Verification items for this drawing (mm, ordinates from the low corner). A direction names the side the tool comes from. Round coordinates to 2 decimals unless told otherwise and drop trailing zeros. Order: outer loops, then holes, each group sorted by start corner. A loop starts at its lowest first (then second) coordinate and runs counter-clockwise, first axis right, second up. Notation, with made-up numbers: M -27,27 L 5,27 A30 cw 5,62 Z; hole C 17.25,87 d2. An arc over 180 degrees is marked long. Return JSON: item names as keys, results as strings. Group by question number.
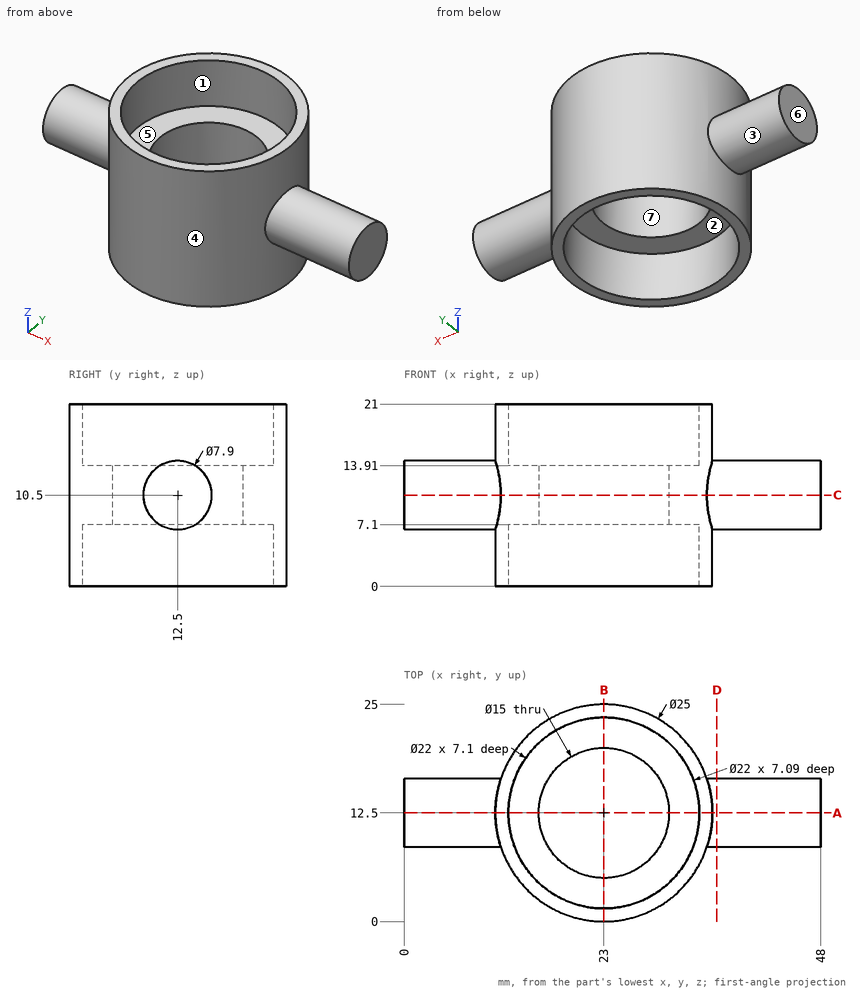
Q1. Section check A-A on y = 12.5. Record the cut outline in (x, z).
Q2. Section check C-C on z = 10.5. Record the cut outline in (x, y).
Q3. Material ranges on line 1 along Y through (x, z) = (23, 18.5); line 2 along Y through (x, z) = (23, 9.5); line 3 along Z through (x, y) = (17, 7), recorded low to high.
Q4. Section check B-B on x = 23. Record the cut outline in (y, z).
Q5. Depth check by flat-ended pin: pin 1 Ø4 at (y, z) = (20, 18.5) entering from +X (3 decimals); pin 2 Ø3 at (x, y) = (39, 13.5) entering from +Z; pin 3 Ø3 at (y, z) = (21, 15) entering from +X. Enter the tip coordinate at first touch or a pass-through.
Q6. Release check for a two-part mould opening along X. For the marked faces 4, 5, 6 and 7 record: +X half, -X half, draft (parallel to the pull), parting line (faces both ways), or undercut.
Q7. Section check D-D on x = 36. Record the cut outline in (y, z).
Q8. Set-up check for the marked faces 1, 2 and 3: record each of +Z, -Z, +X, -X, +Y, -Y from which the full face is reachable in a straight line by a thin tool's end or side.
Geometry check:
{
 "1": {"outline": "M 0,6.55 L 10.5,6.55 L 10.5,0 L 12,0 L 12,7.1 L 15.5,7.1 L 15.5,13.91 L 12,13.91 L 12,21 L 10.5,21 L 10.5,14.45 L 0,14.45 Z; M 30.5,7.1 L 34,7.1 L 34,0 L 35.5,0 L 35.5,6.55 L 48,6.55 L 48,14.45 L 35.5,14.45 L 35.5,21 L 34,21 L 34,13.91 L 30.5,13.91 Z"},
 "2": {"outline": "M 0,8.55 L 11.14,8.55 A12.5 ccw 34.86,8.55 L 48,8.55 L 48,16.45 L 34.86,16.45 A12.5 ccw 11.14,16.45 L 0,16.45 Z; hole C 23,12.5 d15"},
 "3": {"line 1": "y = 0 to 1.5, 23.5 to 25", "line 2": "y = 0 to 5, 20 to 25", "line 3": "z = 7.1 to 13.91"},
 "4": {"outline": "M 0,0 L 1.5,0 L 1.5,7.1 L 5,7.1 L 5,13.91 L 1.5,13.91 L 1.5,21 L 0,21 Z; M 20,7.1 L 23.5,7.1 L 23.5,0 L 25,0 L 25,21 L 23.5,21 L 23.5,13.91 L 20,13.91 Z"},
 "5": {"pin 1": "stops at x = 34.225", "pin 2": "stops at z = 14.45", "pin 3": "stops at x = 33.36"},
 "6": {"face 4": "parting line", "face 5": "undercut", "face 6": "-X half", "face 7": "undercut"},
 "7": {"outline": "C 12.5,10.5 d7.9"},
 "8": {"face 1": "+Z", "face 2": "-Z", "face 3": "-X"}
}
